Here's how the part is built. I have some questions about the finished solid (model axes, mm). Face numbers are marked on the shaded views. Round coordinates to 2 decimals unless told otherwise and drop trailing zeros. Write each loop counter-clockwise with the first axis right and the second up, starting at its lowest first coordinate (ties: lowest second). Pieces come first, ordered by that corner, then holes. Notation, with made-up numbers: (-9, 37.25) -> (9, 37.25) arc R9 ccw to (9, 45.25) -> close; hole circle Ø7 at (56.25, -25). An arc over 180 degrees is marked (long way). Put each result on its own line as item: value. Start each with the question number.
1. We'd pull the mould along Y, two halves only. Please class the marked faces 1 and 2: +Y half, -Y half, draft (parallel to the pull), parting line (faces both ways), or undercut.
2. I need wall thicknesses on probe 1 along Y at (x, z) = (0, 79.5); probe 2 along Y at (x, z) = (0, 45); probe 3 along X at (y, z) = (-5.5, 101). Which ranges of each line are inside material? Lowest first, please. Write a range as from..to.
3. Suppose I cut it at D-D (x = -12.5). Please give me the cut outline in (y, z), then the cut area to 3 significant figures.
4. For pin 1 (8 mm diameter, centred on x = -22.5, z = 45, fed in from +Y); pin 2 (5 mm diameter, centred on x = 0.5, z = 33.5, fed in from +Y); pin 3 (1 mm diameter, centred on y = -12, z = 63, fed in from +X); pin 4 (2 mm diameter, centred on x = -21, y = 10.5, fed in from -Z), each with a flat end and sliding along its axis, tell me the tip position at first contact or that it passes through.
5. Suppose I cut it at C-C (y = 9). Please give me the cut outline in (x, z), then the cut area to 3 significant figures.
6. Suppose I cut it at A-A (x = 11.5). Please give me the cut outline in (y, z), then the cut area to 3 significant figures.
7. Suppose I cut it at B-B (z = 116). Please give me the cut outline in (x, y), then the cut area to 3 significant figures.
```python
from build123d import *

# Parameters (mm, degrees)
CROQUIS1_R                               = 31
CROQUIS1_R_2                             = 25
SALIENTE_EXTRUIR1_DEPTH                  = 130
CROQUIS3_R                               = 29
CORTAR_EXTRUIR1_DEPTH                    = 29.05
SALIENTE_EXTRUIR2_REACH                  = 139.193
SALIENTE_EXTRUIR2_END_RADIUS             = 25
SALIENTE_EXTRUIR2_DIRECTION_2_REACH      = 139.193
SALIENTE_EXTRUIR2_DIRECTION_2_END_RADIUS = 25
CROQUIS6_R                               = 2.5
SALIENTE_EXTRUIR3_DEPTH                  = 20


with BuildPart() as part:
    # Croquis1 → Saliente-Extruir1 (new body)
    with BuildSketch(Plane.XY):
        Circle(CROQUIS1_R)
        Circle(CROQUIS1_R_2, mode=Mode.SUBTRACT)
    extrude(amount=SALIENTE_EXTRUIR1_DEPTH)

    # Croquis3 → Cortar-Extruir1 (cut)
    with BuildSketch(Plane(origin=(0, 40, 0), x_dir=(1, 0, 0), z_dir=(0, 1, 0))):
        with Locations(Location((0, -41, 0), (0, 0, 270))):
            Circle(CROQUIS3_R)
    extrude(amount=-CORTAR_EXTRUIR1_DEPTH, mode=Mode.SUBTRACT)

    # Saliente-Extruir2: up to this cylinder (the profile starts inside it)
    saliente_extruir2_end = Plane(origin=(0, 0, 126.111111), z_dir=(0, 0, -1)) * Cylinder(SALIENTE_EXTRUIR2_END_RADIUS, 329.386, mode=Mode.PRIVATE)
    # Croquis5 → Saliente-Extruir2 (add, up to the surface)
    with BuildSketch(Plane(origin=(0, 0, 0), x_dir=(1, 0, 0), z_dir=(0, 1, 0)), mode=Mode.PRIVATE) as saliente_extruir2_sk1:
        Polygon((-2.5, -130), (2.5, -130), (2.5, -125), (0, -120), (-2.5, -125), align=None)
    saliente_extruir2_tool1 = extrude(saliente_extruir2_sk1.sketch, amount=SALIENTE_EXTRUIR2_REACH, mode=Mode.PRIVATE) & saliente_extruir2_end
    add(saliente_extruir2_tool1.solids().sort_by_distance((0, 0, 126.111111))[0])

    # Saliente-Extruir2 direction 2: up to this cylinder (the profile starts inside it)
    saliente_extruir2_direction_2_end = Plane(origin=(0, 0, 126.111111), z_dir=(0, 0, -1)) * Cylinder(SALIENTE_EXTRUIR2_DIRECTION_2_END_RADIUS, 329.386, mode=Mode.PRIVATE)
    # Croquis5 → Saliente-Extruir2 direction 2 (add, up to the surface)
    with BuildSketch(Plane(origin=(0, 0, 0), x_dir=(1, 0, 0), z_dir=(0, 1, 0)), mode=Mode.PRIVATE) as saliente_extruir2_direction_2_sk1:
        Polygon((-2.5, -130), (2.5, -130), (2.5, -125), (0, -120), (-2.5, -125), align=None)
    saliente_extruir2_direction_2_tool1 = extrude(saliente_extruir2_direction_2_sk1.sketch, amount=-SALIENTE_EXTRUIR2_DIRECTION_2_REACH, mode=Mode.PRIVATE) & saliente_extruir2_direction_2_end
    add(saliente_extruir2_direction_2_tool1.solids().sort_by_distance((0, 0, 126.111111))[0])

    # Croquis6 → Saliente-Extruir3 (add)
    with BuildSketch(Plane.XY.offset(130)):
        Circle(CROQUIS6_R)
    extrude(amount=-SALIENTE_EXTRUIR3_DEPTH)


solid = part.part
```
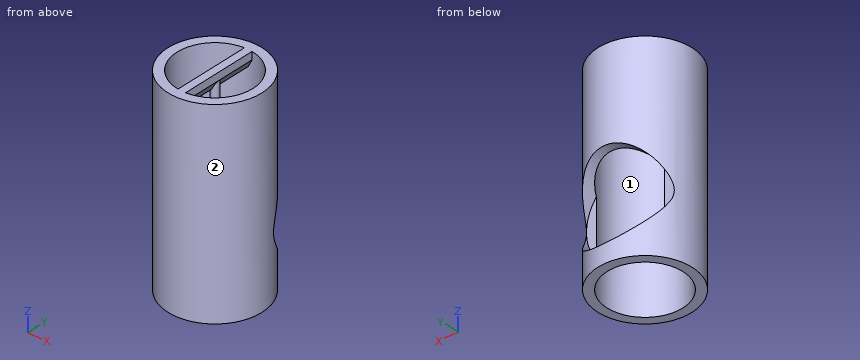
Verdict:
1. face 1: undercut
1. face 2: parting line
2. probe 1: y = -31..-25, 25..31
2. probe 2: y = -31..-25
2. probe 3: x = -30.51..-24.39, 24.39..30.51
3. outline: (-28.37, 0) -> (-21.65, 0) -> (-21.65, 130) -> (-28.37, 130) -> close; (21.65, 0) -> (28.37, 0) -> (28.37, 14.83) -> (21.65, 14.83) -> close; (21.65, 67.17) -> (28.37, 67.17) -> (28.37, 130) -> (21.65, 130) -> close
3. area: 1,390 mm^2
4. pin 1: stops at y = 10.95
4. pin 2: stops at y = -24.82
4. pin 3: stops at x = 28.79
4. pin 4: passes through
5. outline: (-29.66, 0) -> (-23.32, 0) -> (-23.32, 130) -> (-29.66, 130) -> close; (-2.5, 125) -> (0, 120) -> (2.5, 125) -> (2.5, 130) -> (-2.5, 130) -> close; (23.32, 0) -> (29.66, 0) -> (29.66, 130) -> (23.32, 130) -> close
5. area: 1,690 mm^2
6. outline: (-28.79, 0) -> (-22.2, 0) -> (-22.2, 130) -> (-28.79, 130) -> close; (22.2, 0) -> (28.79, 0) -> (28.79, 14.38) -> (22.2, 14.38) -> close; (22.2, 67.62) -> (28.79, 67.62) -> (28.79, 130) -> (22.2, 130) -> close
6. area: 1,360 mm^2
7. outline: circle Ø62 at (0, 0); circle Ø5 at (0, 0); hole circle Ø50 at (0, 0)
7. area: 1,080 mm^2
